from build123d import *

# Parameters (mm, degrees)
BOSS_EXTRUDE1_DEPTH = 15.875
SKETCH3_R           = 12.7
BOSS_EXTRUDE2_DEPTH = 12.7
SKETCH4_R           = 9.525
CUT_EXTRUDE1_DEPTH  = 42.481266827


with BuildPart() as part:
    # Sketch1 → Boss-Extrude1 (new body)
    with BuildSketch(Plane(origin=(0, 0, 0), x_dir=(1, 0, 0), z_dir=(0, 1, 0))):
        Polygon((19.685, -11.365140049), (19.685, 11.365140049), (0, 22.730280098), (-19.685, 11.365140049), (-19.685, -11.365140049), (0, -22.730280098), align=None)
    extrude(amount=BOSS_EXTRUDE1_DEPTH)

    # Sketch2 → Cut-Revolve1 (revolve, cut)
    with BuildSketch(Plane(origin=(0, 0, 0), x_dir=(0, 0, -1), z_dir=(1, 0, 0))):
        with BuildLine():
            Line((22.730280098, 0), (28.475559527, 0))
            Line((28.475559527, 0), (28.475559527, 20.473836959))
            Line((28.475559527, 20.473836959), (11.365140049, 20.473836959))
            Line((11.365140049, 20.473836959), (11.365140049, 15.875))
            Line((11.365140049, 15.875), (15.110280098, 15.875))
            ThreePointArc((15.110280098, 15.875), (20.498433771, 13.643153673), (22.730280098, 8.255))
            Line((22.730280098, 8.255), (22.730280098, 0))
        make_face()
    revolve(axis=Axis((0, 0, 0), (0, 1, 0)), mode=Mode.SUBTRACT)

    # Sketch3 → Boss-Extrude2 (add)
    with BuildSketch(Plane(origin=(0, 15.875, 0), x_dir=(1, 0, 0), z_dir=(0, 1, 0))):
        with Locations(Location((0, 0, 0), (0, 0, 270))):
            Circle(SKETCH3_R)
    extrude(amount=BOSS_EXTRUDE2_DEPTH)

    # Sketch4 → Cut-Extrude1 (cut, through all)
    with BuildSketch(Plane(origin=(0, 28.575, 0), x_dir=(1, 0, 0), z_dir=(0, 1, 0))):
        with Locations(Location((0, 0, 0), (0, 0, 270))):
            Circle(SKETCH4_R)
    extrude(amount=-CUT_EXTRUDE1_DEPTH, mode=Mode.SUBTRACT)


solid = part.part
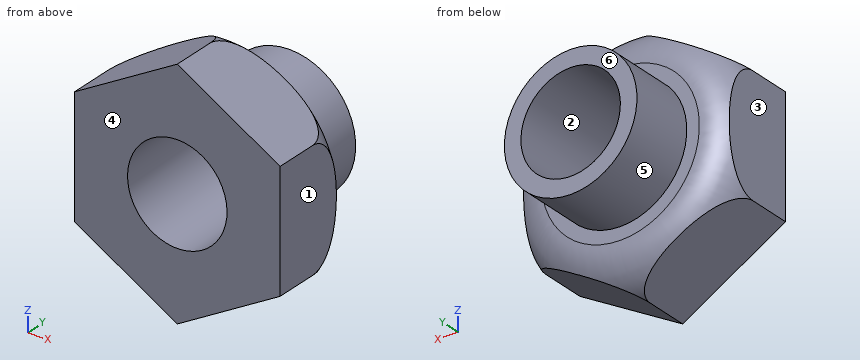
Verification items for the finished model (mm, model axes). Face numbers are marked on the shaded views. A direction names the side the tool comes from. Give positions to 0.01 mm unless a question says otherwise; leave off trailing zeros. Write each loop counter-clockwise with the first axis right and the second up, starting at its lowest first coordinate (ties: lowest second). Pieces come first, ordered by that corner, then holes.
(1) Mould release check, pull along X, two halves, no side actions. Record for the marked faces 1, 2, 3 and 4: +X half, -X half, draft (parallel to the pull), parting line (faces both ways), or undercut.
(2) Access from +Z, -Z, +X, -X, +Y, -Y to the whole of each face (thin tool, end or side, straight path). Record for the marked faces 5 and 6.
(3) Cross-section at A-A (z = 0). Enter the section's corners in (x, y) (3 decimals).
(4) Gauge pin test, flat end, axial feed: pin 1 (1 mm diameter, centred on x = -13.5, z = -0.5, fed in from -Y). Record the tip position at first contact, or that the pin passes through.
(5) Material ranges on line 1 (Z direction, x = 0.5, y = 16.5); line 2 (X direction, y = 13.5, z = 0) (3 decimals); line 3 (X direction, y = 20.5, z = 0) (3 decimals), recorded low to high.
(6) Cross-section at B-B (y = 2). Enter the section's corners in (x, z) (3 decimals).
(7) Cross-section at C-C (y = 11.5). Enter the section's corners in (x, z) (3 decimals).
(8) Cross-section at D-D (y = 22.75). Enter the section's corners in (x, z) (3 decimals), plus the area to 3 significant figures.
Worked out:
1. face 1: +X half
1. face 2: undercut
1. face 3: -X half
1. face 4: draft
2. face 5: +Y
2. face 6: +Z, -Z, +X, -X, +Y
3. outline: (-19.685, 0) - (-9.525, 0) - (-9.525, 28.575) - (-12.7, 28.575) - (-12.7, 15.875) - (-15.11, 15.875) arc R7.62 ccw to (-19.685, 14.349) - close; (9.525, 0) - (19.685, 0) - (19.685, 14.349) arc R7.62 ccw to (15.11, 15.875) - (12.7, 15.875) - (12.7, 28.575) - (9.525, 28.575) - close
4. pin 1: stops at y = 0
5. line 1: z = -12.69 to -9.51, 9.51 to 12.69
5. line 2: x = -19.685 to -9.525, 9.525 to 19.685
5. line 3: x = -12.7 to -9.525, 9.525 to 12.7
6. outline: (-19.685, -11.365) - (0, -22.73) - (19.685, -11.365) - (19.685, 11.365) - (0, 22.73) - (-19.685, 11.365) - close; hole circle Ø19.05 at (0, 0)
7. outline: (-19.685, -9.834) arc R22.005 ccw to (-18.359, -12.131) - (-1.326, -21.965) arc R22.005 ccw to (1.326, -21.965) - (18.359, -12.131) arc R22.005 ccw to (19.685, -9.834) - (19.685, 9.834) arc R22.005 ccw to (18.359, 12.131) - (1.326, 21.965) arc R22.005 ccw to (-1.326, 21.965) - (-18.359, 12.131) arc R22.005 ccw to (-19.685, 9.834) - close; hole circle Ø19.05 at (0, 0)
8. outline: circle Ø25.4 at (0, 0); hole circle Ø19.05 at (0, 0)
8. area: 222 mm2
